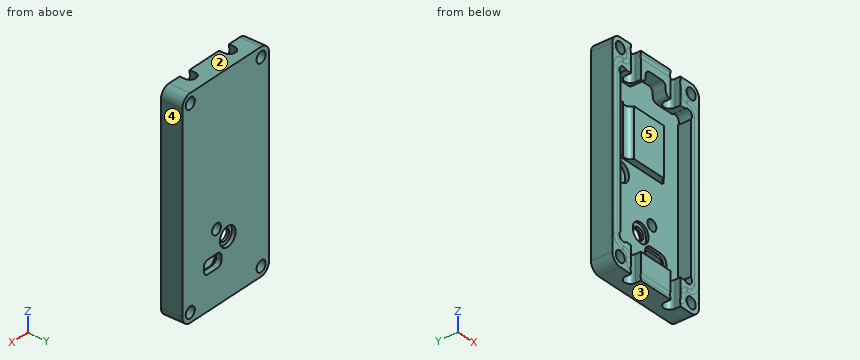
```python
from build123d import *

# Parameters (mm, degrees)
SKETCH1_W             = 34.925
SKETCH1_H             = 69.85
BOSS_EXTRUDE1_DEPTH   = 7.112
FILLET1_R             = 3.175
SKETCH8_R             = 2.38125
BOSS_EXTRUDE2_DEPTH   = 7.112
SKETCH9_R             = 2.0193
CUT_EXTRUDE6_DEPTH    = 8.112
SKETCH12_W            = 28.25399988
SKETCH12_H            = 52.253999886
CUT_EXTRUDE8_DEPTH    = 4.318
FILLET2_R             = 1.5875
SKETCH16_W            = 17.272
SKETCH16_H            = 16.002
BOSS_EXTRUDE3_DEPTH   = 2.0574
CUT_EXTRUDE10_DEPTH   = 70.85
F_6_CLEARANCE_HOLE1_D = 3.6576
SKETCH36_W            = 8.08260004
SKETCH36_H            = 4.035500057
CUT_EXTRUDE17_DEPTH   = 4.318
FILLET3_R             = 1.5875
CUT_EXTRUDE18_DEPTH   = 3.794
SKETCH38_R            = 3.175
CUT_EXTRUDE19_DEPTH   = 1.2446
SKETCH39_R            = 1.778
CUT_EXTRUDE20_DEPTH   = 2.8956
SKETCH40_R            = 1.5875
CUT_EXTRUDE21_DEPTH   = 5.3180001
SKETCH41_R            = 3.175
CUT_EXTRUDE22_DEPTH   = 1.27
SKETCH42_R            = 3.175
CUT_EXTRUDE23_DEPTH   = 0.762
CUT_EXTRUDE24_DEPTH   = 1.016


with BuildPart() as part:
    # Sketch1 → Boss-Extrude1 (new body)
    with BuildSketch(Plane(origin=(0, 0, 0), x_dir=(1, 0, 0), z_dir=(0, 1, 0))):
        Rectangle(SKETCH1_W, SKETCH1_H)
    extrude(amount=BOSS_EXTRUDE1_DEPTH)

    # Fillet1
    fillet1_edges = [part.edges().sort_by_distance(p)[0] for p in [
        (17.4625, 3.556, 34.925),
        (-17.4625, 3.556, 34.925),
        (-17.4625, 3.556, -34.925),
        (17.4625, 3.556, -34.925),
    ]]
    fillet(fillet1_edges, radius=FILLET1_R)

    # Sketch8 → Boss-Extrude2 (add)
    with BuildSketch(Plane(origin=(0, 0, 0), x_dir=(1, 0, 0), z_dir=(0, 1, 0))):
        with Locations((-1.2573, 21.6662)):
            Circle(SKETCH8_R)
    extrude(amount=BOSS_EXTRUDE2_DEPTH)

    # Sketch9 → Cut-Extrude6 (cut, through all)
    with BuildSketch(Plane(origin=(0, 7.112, 0), x_dir=(1, 0, 0), z_dir=(0, 1, 0))):
        with Locations((-0.8255, 16.129)):
            Circle(SKETCH9_R)
    extrude(amount=-CUT_EXTRUDE6_DEPTH, mode=Mode.SUBTRACT)

    # Sketch12 → Cut-Extrude8 (cut)
    with BuildSketch(Plane.XZ):
        Rectangle(SKETCH12_W, SKETCH12_H)
    extrude(amount=-CUT_EXTRUDE8_DEPTH, mode=Mode.SUBTRACT)

    # Fillet2
    fillet2_edges = [part.edges().sort_by_distance(p)[0] for p in [
        (-14.12699994, 2.159, 26.126999943),
        (14.12699994, 2.159, 26.126999943),
        (14.12699994, 2.159, -26.126999943),
        (-14.12699994, 2.159, -26.126999943),
    ]]
    fillet(fillet2_edges, radius=FILLET2_R)

    # Sketch16 → Boss-Extrude3 (add)
    with BuildSketch(Plane.XZ.offset(-4.318)):
        with Locations((-0.847000084, 10.947000013)):
            Rectangle(SKETCH16_W, SKETCH16_H)
    extrude(amount=BOSS_EXTRUDE3_DEPTH)

    # Cut-Sweep1: sweep along a path in Sketch31
    with BuildLine(Plane.XZ) as cut_sweep1_path:
        Line((-12.7, 28.575), (-13.096875, 28.575))
        ThreePointArc((-13.096875, 28.575), (-15.34193903, 27.64506403), (-16.271875, 25.4))
        Line((-16.271875, 25.4), (-16.271875, -25.4))
        ThreePointArc((-16.271875, -25.4), (-15.34193903, -27.64506403), (-13.096875, -28.575))
        Line((-13.096875, -28.575), (-12.7, -28.575))
        ThreePointArc((-12.7, -28.575), (-11.577467985, -29.039967985), (-11.1125, -30.1625))
        Line((-11.1125, -30.1625), (-11.1125, -31.75))
        ThreePointArc((-11.1125, -31.75), (-10.647532015, -32.872532015), (-9.525, -33.3375))
        Line((-9.525, -33.3375), (9.525, -33.3375))
        ThreePointArc((9.525, -33.3375), (10.647532015, -32.872532015), (11.1125, -31.75))
        Line((11.1125, -31.75), (11.1125, -30.1625))
        ThreePointArc((11.1125, -30.1625), (11.577467985, -29.039967985), (12.7, -28.575))
        Line((12.7, -28.575), (13.096875, -28.575))
        ThreePointArc((13.096875, -28.575), (15.34193903, -27.64506403), (16.271875, -25.4))
        Line((16.271875, -25.4), (16.271875, 25.4))
        ThreePointArc((16.271875, 25.4), (15.34193903, 27.64506403), (13.096875, 28.575))
        Line((13.096875, 28.575), (12.7, 28.575))
        ThreePointArc((12.7, 28.575), (11.577467985, 29.039967985), (11.1125, 30.1625))
        Line((11.1125, 30.1625), (11.1125, 31.75))
        ThreePointArc((11.1125, 31.75), (10.647532015, 32.872532015), (9.525, 33.3375))
        Line((9.525, 33.3375), (-9.525, 33.3375))
        ThreePointArc((-9.525, 33.3375), (-10.647532015, 32.872532015), (-11.1125, 31.75))
        Line((-11.1125, 31.75), (-11.1125, 30.1625))
        ThreePointArc((-11.1125, 30.1625), (-11.577467985, 29.039967985), (-12.7, 28.575))
    # Sketch32 → Cut-Sweep1 (sweep, cut)
    with BuildSketch(Plane(origin=(0, 0, 0), x_dir=(0, 0, -1), z_dir=(1, 0, 0))):
        with BuildLine():
            Line((-34.067501479, 0), (-32.607498521, 0))
            ThreePointArc((-32.607498521, 0), (-33.3375, 0.1778), (-34.067501479, 0))
        make_face()
    sweep(path=cut_sweep1_path.line, mode=Mode.SUBTRACT)

    # Sketch15 → Cut-Extrude10 (cut, through all)
    with BuildSketch(Plane(origin=(0, 0, -34.925), x_dir=(-1, 0, 0), z_dir=(0, 0, -1))):
        with BuildLine():
            Line((-5.94630002, 0), (-5.94630002, 1.80000002))
            ThreePointArc((-5.94630002, 1.80000002), (-7.94630002, 3.80000002), (-9.94630002, 1.80000002))
            Line((-9.94630002, 1.80000002), (-9.94630002, 0))
            ThreePointArc((-9.94630002, 0), (-7.94630002, -2), (-5.94630002, 0))
        make_face()
        with BuildLine():
            Line((9.9375, 0), (9.9375, 1.80000002))
            ThreePointArc((9.9375, 1.80000002), (7.9375, 3.80000002), (5.9375, 1.80000002))
            Line((5.9375, 1.80000002), (5.9375, 0))
            ThreePointArc((5.9375, 0), (7.9375, -2), (9.9375, 0))
        make_face()
    extrude(amount=-CUT_EXTRUDE10_DEPTH, mode=Mode.SUBTRACT)

    # #6 Clearance Hole1 (through all)
    with Locations(Plane(origin=(0, 7.112, 0), x_dir=(1, 0, 0), z_dir=(0, 1, 0))):
        with Locations((-14.2875, -31.75), (-14.2875, 31.75), (14.2875, 31.75), (14.2875, -31.75)):
            Hole(F_6_CLEARANCE_HOLE1_D / 2)

    # Sketch36 → Cut-Extrude17 (cut)
    with BuildSketch(Plane.XZ):
        with Locations((0, 28.144749972)):
            Rectangle(SKETCH36_W, SKETCH36_H)
    extrude(amount=-CUT_EXTRUDE17_DEPTH, mode=Mode.SUBTRACT)

    # Fillet3
    fillet3_edges = [part.edges().sort_by_distance(p)[0] for p in [
        (4.04130002, 2.159, 30.1625),
        (4.04130002, 2.159, 26.126999943),
        (-4.04130002, 2.159, 26.126999943),
        (-4.04130002, 2.159, 30.1625),
    ]]
    fillet(fillet3_edges, radius=FILLET3_R)

    # Sketch37 → Cut-Extrude18 (cut, through all)
    with BuildSketch(Plane.XZ.offset(-4.318)):
        with BuildLine():
            Line((7.187867925, -23.670967928), (3.336931955, -23.670967928))
            ThreePointArc((3.336931955, -23.670967928), (2.21439994, -23.205999943), (1.749431955, -22.083467928))
            Line((1.749431955, -22.083467928), (1.749431955, -20.772531958))
            ThreePointArc((1.749431955, -20.772531958), (2.21439994, -19.649999943), (3.336931955, -19.185031958))
            Line((3.336931955, -19.185031958), (7.187867925, -19.185031958))
            ThreePointArc((7.187867925, -19.185031958), (8.31039994, -19.649999943), (8.775367925, -20.772531958))
            Line((8.775367925, -20.772531958), (8.775367925, -22.083467928))
            ThreePointArc((8.775367925, -22.083467928), (8.31039994, -23.205999943), (7.187867925, -23.670967928))
        make_face()
    extrude(amount=-CUT_EXTRUDE18_DEPTH, mode=Mode.SUBTRACT)

    # Sketch38 → Cut-Extrude19 (cut)
    with BuildSketch(Plane.XZ.offset(-4.318)):
        with Locations((-8.72949994, -1.425499943)):
            Circle(SKETCH38_R)
    extrude(amount=-CUT_EXTRUDE19_DEPTH, mode=Mode.SUBTRACT)

    # Sketch39 → Cut-Extrude20 (cut)
    with BuildSketch(Plane.XZ.offset(-4.318)):
        with Locations((3.71299994, -11.648999943)):
            Circle(SKETCH39_R)
    extrude(amount=-CUT_EXTRUDE20_DEPTH, mode=Mode.SUBTRACT)

    # Sketch40 → Cut-Extrude21 (cut, through all)
    with BuildSketch(Plane.XZ.offset(-4.318)):
        with Locations((13.004467925, 25.004467928)):
            Circle(SKETCH40_R)
        with Locations((13.004467925, -25.004467928)):
            Circle(SKETCH40_R)
        with Locations((-13.004467925, -25.004467928)):
            Circle(SKETCH40_R)
        with Locations((-13.004467925, 25.004467928)):
            Circle(SKETCH40_R)
    extrude(amount=CUT_EXTRUDE21_DEPTH, mode=Mode.SUBTRACT)

    # Sketch41 → Cut-Extrude22 (cut)
    with BuildSketch(Plane(origin=(0, 7.112, 0), x_dir=(1, 0, 0), z_dir=(0, 1, 0))):
        with Locations((-0.8255, 16.129)):
            Circle(SKETCH41_R)
    extrude(amount=-CUT_EXTRUDE22_DEPTH, mode=Mode.SUBTRACT)

    # Sketch42 → Cut-Extrude23 (cut)
    with BuildSketch(Plane.XZ.offset(-4.318)):
        with Locations((-0.8255, -16.129)):
            Circle(SKETCH42_R)
    extrude(amount=-CUT_EXTRUDE23_DEPTH, mode=Mode.SUBTRACT)

    # Sketch43 → Cut-Extrude24 (cut)
    with BuildSketch(Plane.XZ.offset(-4.318)):
        with BuildLine():
            Line((0.987431955, -20.772531958), (0.987431955, -22.083467928))
            ThreePointArc((0.987431955, -22.083467928), (1.675584573, -23.74481531), (3.336931955, -24.432967928))
            Line((3.336931955, -24.432967928), (7.187867925, -24.432967928))
            ThreePointArc((7.187867925, -24.432967928), (8.849215307, -23.74481531), (9.537367925, -22.083467928))
            Line((9.537367925, -22.083467928), (9.537367925, -20.772531958))
            ThreePointArc((9.537367925, -20.772531958), (8.849215307, -19.111184576), (7.187867925, -18.423031958))
            Line((7.187867925, -18.423031958), (3.336931955, -18.423031958))
            ThreePointArc((3.336931955, -18.423031958), (1.675584573, -19.111184576), (0.987431955, -20.772531958))
        make_face()
    extrude(amount=-CUT_EXTRUDE24_DEPTH, mode=Mode.SUBTRACT)


solid = part.part
```
Design review of the part built by this model. Coordinates are the model's own, in mm. Face numbers are marked on the shaded views. A direction names the side the tool comes from. Coordinates: 2 decimals unless noted, no trailing zeros. Loops run counter-clockwise (first coordinate to the right, second up) from the corner with the lowest first, then second, coordinate; pieces in that order, holes last. Notation, with made-up numbers: M 27.5,12.25 L 47.5,12.25 A11 cw 47.5,33.25 Z; hole C -39.5,40 d8. An arc over 180 degrees is marked long. One line per question, with ' | ' between items.
(1) We need section B-B (z = 15.5). Give the boundary of the cut face in (x, y) (1 decimal).
Filled in:
outline: M -17.5,0 L -17,0 A1.6 cw -15.5,0 L -14.1,0 L -14.1,4.3 L -9.5,4.3 L -9.5,3.1 A2 cw -6,2.3 L 6,2.3 A2 cw 7.8,3.8 L 7.8,4.3 L 14.1,4.3 L 14.1,0 L 15.5,0 A1.6 cw 17,0 L 17.5,0 L 17.5,7.1 L -17.5,7.1 Z
(2) Machinability: for the marked faces 4 and 5, which of the approach directions +Z, -Z, +X, -X, +Y, -Y give a long, thin tool a straight path to every point of the face, cutting with its end or side? Answer none if there is none.
Filled in:
face 4: +Z, -Z, +X, +Y, -Y | face 5: -Y
(3) We need section A-A (z = -10.5). Give the boundary of the cut face in (x, y) (1 decimal).
Filled in:
outline: M -17.5,0 L -17,0 A1.6 cw -15.5,0 L -14.1,0 L -14.1,4.3 L 2.4,4.3 L 2.4,7.1 L -17.5,7.1 Z; M 5.1,4.3 L 14.1,4.3 L 14.1,0 L 15.5,0 A1.6 cw 17,0 L 17.5,0 L 17.5,7.1 L 5.1,7.1 Z
(4) For pin 1 Ø5 at (x, z) = (-8.5, -2) entering from -Y; pin 2 Ø0.9 at (y, z) = (1.5, -32.5) entering from -X; pin 3 Ø5.5 at (x, z) = (-0.83, -16.13) entering from -Y, all flat-tipped, find the tip position at first contact; note any pin that passes through.
Filled in:
pin 1: stops at y = 5.56 | pin 2: stops at x = -17.45 | pin 3: stops at y = 5.08
(5) Draft analysis for pull direction Z (two halves, no side actions). For the marked faces 1, 2 and 3, state which applies: released by +Z, released by -Z, zero draft, split by the parting line, or undercut.
Filled in:
face 1: undercut | face 2: released by +Z | face 3: released by -Z
(6) We need section C-C (x = -8). Give the boundary of the cut face in (y, z) (3 decimals), and give its area (3 significant figures).
Filled in:
outline: M 3.799,-34.925 L 7.112,-34.925 L 7.112,34.925 L 3.799,34.925 L 3.799,26.127 L 4.318,26.127 L 4.318,18.948 L 3.799,18.948 L 3.799,2.946 L 4.318,2.946 L 4.318,1.665 L 5.563,1.665 L 5.563,-4.516 L 4.318,-4.516 L 4.318,-26.127 L 3.799,-26.127 Z | area: 205 mm^2
(7) Wall thickness on probe 1 along X at (y, z) = (4, 31.75); probe 2 along Z at (x, y) = (7, 4) (3 decimals); probe 3 along Z at (x, y) = (13, 3) (3 decimals): over which ranges is each line inside the solid? List them lowest first.
Filled in:
probe 1: x = -17.46 to -16.12, -12.46 to 12.46, 16.12 to 17.46 | probe 2: z = -34.925 to -26.127, 2.946 to 18.948, 26.127 to 34.925 | probe 3: z = -34.925 to -33.049, -30.451 to -26.592, 26.592 to 30.451, 33.049 to 34.925
